from build123d import *

# Parameters (mm, degrees)
EXTRUDE_THIN1_DEPTH = 25
CUT_EXTRUDE1_REACH  = 95.408
CUT_EXTRUDE2_REACH  = 95.248
SKETCH4_R           = 15
EXTRUDE_THIN2_DEPTH = 44
FILLET2_R           = 18
CUT_EXTRUDE4_REACH  = 95.113
SKETCH8_R           = 5
CUT_EXTRUDE9_DEPTH  = 14.666666666


with BuildPart() as part:
    # Sketch1 → Extrude-Thin1 (new, symmetric)
    with BuildSketch(Plane.XY):
        Polygon((-45.961940777, -45.961940777), (0, 0), (70, 0), (70, -15), (6.213203436, -15), (-35.355339059, -56.568542495), align=None)
    extrude(amount=EXTRUDE_THIN1_DEPTH, both=True)

    # Sketch3 → Cut-Extrude1 (cut, up to next)
    with BuildSketch(Plane(origin=(0, 0, 0), x_dir=(0, 0, 1), z_dir=(-0.707106781186544, 0.7071067811865511, 0)), mode=Mode.PRIVATE) as cut_extrude1_sk1:
        with BuildLine():
            Line((-25, -39.625598043), (-40.613417223, -39.625598043))
            Line((-40.613417223, -39.625598043), (-40.613417223, -78.57107129))
            Line((-40.613417223, -78.57107129), (38.176612189, -78.57107129))
            Line((38.176612189, -78.57107129), (38.176612189, -39.625598043))
            Line((38.176612189, -39.625598043), (25, -39.625598043))
            ThreePointArc((25, -39.625598043), (0, -64.625598043), (-25, -39.625598043))
        make_face()
    cut_extrude1_tool1 = extrude(cut_extrude1_sk1.sketch, amount=-CUT_EXTRUDE1_REACH, mode=Mode.PRIVATE) & part.part
    add(cut_extrude1_tool1.solids().sort_by_distance((-28.641004, -28.641004, -32.806709))[0], mode=Mode.SUBTRACT)

    # Sketch4 → Cut-Extrude2 (cut, up to next)
    with BuildSketch(Plane(origin=(0, 0, 0), x_dir=(0, 0, 1), z_dir=(-0.707106781186544, 0.7071067811865511, 0)), mode=Mode.PRIVATE) as cut_extrude2_sk1:
        with Locations(Location((0, -39.625598043, 0), (0, 0, 270))):
            Circle(SKETCH4_R)
    cut_extrude2_tool1 = extrude(cut_extrude2_sk1.sketch, amount=-CUT_EXTRUDE2_REACH, mode=Mode.PRIVATE) & part.part
    add(cut_extrude2_tool1.solids().sort_by_distance((-28.019529, -28.019529, 0))[0], mode=Mode.SUBTRACT)

    # Sketch6 → Extrude-Thin2 (add)
    with BuildSketch(Plane(origin=(70, 0, 0), x_dir=(0, 0, -1), z_dir=(1, 0, 0))):
        Polygon((19.884546135, -8.860225997), (25, 0), (42.5, 30.310889132), (32.973720558, 35.810889132), (15.473720558, 5.5), (10.358266694, -3.360225997), align=None)
    extrude(amount=-EXTRUDE_THIN2_DEPTH)

    # Fillet2
    fillet2_edges = [part.edges().sort_by_distance(p)[0] for p in [
        (70, 33.060889132, -37.736860279),
    ]]
    fillet(fillet2_edges, radius=FILLET2_R)

    # Sketch8 → Cut-Extrude4 (cut, up to next)
    with BuildSketch(Plane(origin=(0, -5.325317547, -9.223720558), x_dir=(1, 0, 0), z_dir=(0, 0.4999999999999978, 0.86602540378444)), mode=Mode.PRIVATE) as cut_extrude4_sk1:
        with Locations(Location((52.289208075, 30.640066592, 0), (0, 0, 270))):
            Circle(SKETCH8_R)
    cut_extrude4_tool1 = extrude(cut_extrude4_sk1.sketch, amount=-CUT_EXTRUDE4_REACH, mode=Mode.PRIVATE) & part.part
    add(cut_extrude4_tool1.solids().sort_by_distance((52.289208, 21.209758, -24.543754))[0], mode=Mode.SUBTRACT)

    # Sketch10 → Cut-Extrude9 (cut, along a direction that is not the sketch's normal)
    with BuildSketch(Plane(origin=(0, -5.325317547, -9.223720558), x_dir=(1, 0, 0), z_dir=(0, 0.4999999999999978, 0.86602540378444))):
        Polygon((26, 6.149147039), (52, 47.5), (26, 47.5), align=None)
    extrude(amount=-CUT_EXTRUDE9_DEPTH, dir=(0, 0, 1), mode=Mode.SUBTRACT)


solid = part.part
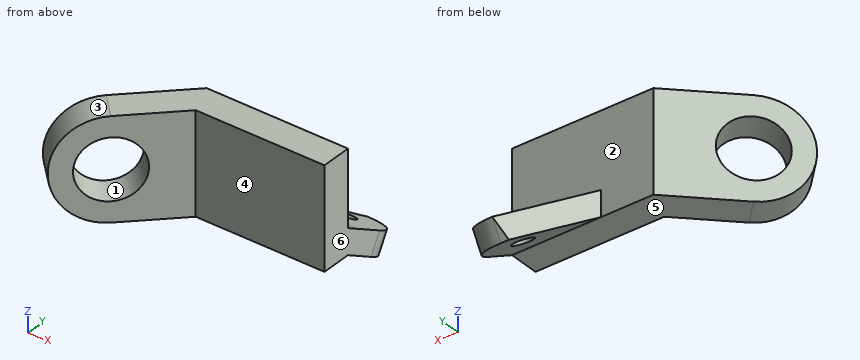
Design review of the part built by this model. Coordinates are the model's own, in mm. Face numbers are marked on the shaded views. A direction names the side the tool comes from. Coordinates: 2 decimals unless noted, no trailing zeros. Order: outer loops, then holes, each group sorted by start corner. A loop starts at its lowest first (then second) coordinate and runs counter-clockwise, first axis right, second up. Notation, with made-up numbers: (4.5, 29.25) -> (38.5, 29.25) arc R12 cw to (38.5, 45.25) -> close; hole circle Ø6 at (-20, 54.25). An arc over 180 degrees is marked (long way). Use one line per item in the form item = value. Start each with the question number.
(1) For the marked faces 4, 5 and 6, list the 3-axis set-ups (+Z, -Z, +X, -X, +Y, -Y) from which the entire face can be reached by the end or side of a thin tool; tool diameter is ignored.
(2) Add section D-D on y = 7.5. State the section outline as (x, z) points.
(3) For probe 1 along Y at (x, z) = (14.5, -3.5); probe 2 along Z at (x, y) = (4, -9.5); probe 3 along X at (y, z) = (-34.5, -16.5), list the stretches that pass through material, from the lowest coordinate up.
(4) Add section A-A on z = -4. State the section outline as (x, y) points.
(5) Insertion check: pin 1 (6 mm diameter, centred on x = -23.5, y = -29, fed in from -Z); pin 2 (12 mm diameter, centred on y = 19.5, z = -10, fed in from +X); pin 3 (15 mm diameter, centred on x = 39, z = 9.5, fed in from -Y); pin 4 (4 mm diameter, centred on x = 6, z = -14, fed in from +Y). Each pin has a flat end and moves straight along its axis. Give the tip position at first contact, or say it passes through.
(6) Add section C-C on z = -19.5. State the section outline as (x, y) points, plus the area to 3 significant figures.
(7) Add section B-B on x = 39.5. State the section outline as (y, z) points.
(8) The part is to be moulded in two halves that separate along Z. For the marked faces 1, 2 and 3, say which applies: +Z half, -Z half, draft (parallel to the pull), parting line (faces both ways), or undercut.
Answer block:
q1.face_4 = +Z, -Z, +X, -Y
q1.face_5 = -Z, +X, -X, -Y
q1.face_6 = +Z, -Z, +X, +Y, -Y
q2.outline = (31.45, -29.33) -> (70, -29.33) -> (70, -16.63) -> (31.45, -16.63) -> close
q3.probe_1 = -15 to 0
q3.probe_2 = -25 to 25
q3.probe_3 = -34.5 to -13.29
q4.outline = (-45.47, -45.47) -> (-34.86, -56.08) -> (-27.64, -48.85) -> (-38.24, -38.24) -> close; (-17.8, -17.8) -> (-7.19, -28.4) -> (6.21, -15) -> (70, -15) -> (70, 0) -> (0, 0) -> close
q5.pin_1 = -25
q5.pin_2 = through
q5.pin_3 = -15
q5.pin_4 = 0
q6.outline = (-39.08, -39.08) -> (-28.48, -49.69) -> (6.21, -15) -> (70, -15) -> (70, 12.47) -> (35.06, 12.47) -> (26, 0) -> (0, 0) -> close
q6.area = 2,280 mm²
q7.outline = (-15, -25) -> (0, -25) -> (18.59, -35.74) -> (18.59, -23.03) -> (0, -12.3) -> (0, 25) -> (-15, 25) -> close
q8.face_1 = undercut
q8.face_2 = draft
q8.face_3 = parting line
